Build history of the part. All positions in model axes, mm. Face numbers are marked on the shaded views. Give positions to 0.01 mm unless a question says otherwise; leave off trailing zeros. Order: outer loops, then holes, each group sorted by start corner. A loop starts at its lowest first (then second) coordinate and runs counter-clockwise, first axis right, second up. Notation, with made-up numbers: M 32.5,73.5 L 67.5,73.5 A28 cw 67.5,95.5 Z; hole C 14,68 d6. An arc over 180 degrees is marked long. One line per item, written item: value. Start each with the question number.
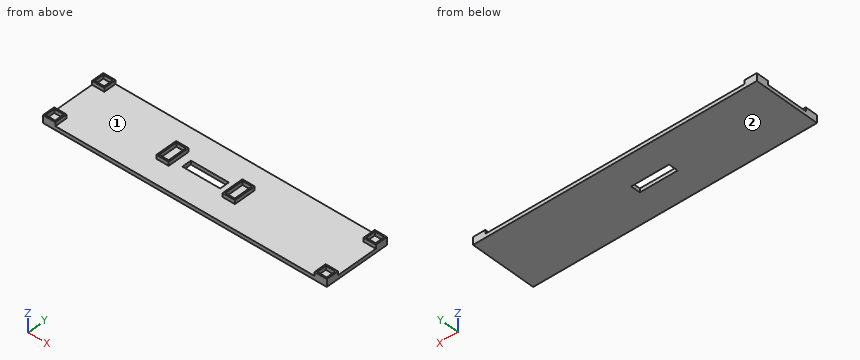
from build123d import *

# Parameters (mm, degrees)
SKICA1_W                 = 150
SKICA1_H                 = 35
P_IDAT_VYSUNUT_M2_DEPTH  = 2
SKICA2_W                 = 6.5
SKICA2_H                 = 11.5
SKICA2_W_2               = 5
SKICA2_H_2               = 10
P_IDAT_VYSUNUT_M3_DEPTH  = 2
SKICA3_W                 = 6.5
SKICA3_H                 = 6.5
SKICA3_W_2               = 5
SKICA3_H_2               = 5
P_IDAT_VYSUNUT_M4_DEPTH  = 2
SKICA4_W                 = 20
SKICA4_H                 = 5
ODEBRAT_VYSUNUT_M1_DEPTH = 2


with BuildPart() as part:
    # Skica1 → Přidat vysunutím2 (new body)
    with BuildSketch(Plane.XY):
        Rectangle(SKICA1_W, SKICA1_H)
    extrude(amount=P_IDAT_VYSUNUT_M2_DEPTH)

    # Skica2 → Přidat vysunutím3 (add)
    with BuildSketch(Plane.XY.offset(2)):
        with Locations((-22.5, 0)):
            Rectangle(SKICA2_W, SKICA2_H)
        with Locations((-22.5, 0)):
            Rectangle(SKICA2_W_2, SKICA2_H_2, mode=Mode.SUBTRACT)
        with Locations((12.5, 0)):
            Rectangle(SKICA2_W, SKICA2_H)
        with Locations((12.5, 0)):
            Rectangle(SKICA2_W_2, SKICA2_H_2, mode=Mode.SUBTRACT)
    extrude(amount=P_IDAT_VYSUNUT_M3_DEPTH)

    # Skica3 → Přidat vysunutím4 (add)
    with BuildSketch(Plane.XY.offset(2)):
        with Locations((-71.75, 14.25)):
            Rectangle(SKICA3_W, SKICA3_H)
        with Locations((-71.75, 14.25)):
            Rectangle(SKICA3_W_2, SKICA3_H_2, mode=Mode.SUBTRACT)
        with Locations((71.75, 14.25)):
            Rectangle(SKICA3_W, SKICA3_H)
        with Locations((71.75, 14.25)):
            Rectangle(SKICA3_W_2, SKICA3_H_2, mode=Mode.SUBTRACT)
        with Locations((-71.75, -14.25)):
            Rectangle(SKICA3_W, SKICA3_H)
        with Locations((-71.75, -14.25)):
            Rectangle(SKICA3_W_2, SKICA3_H_2, mode=Mode.SUBTRACT)
        with Locations((71.75, -14.25)):
            Rectangle(SKICA3_W, SKICA3_H)
        with Locations((71.75, -14.25)):
            Rectangle(SKICA3_W_2, SKICA3_H_2, mode=Mode.SUBTRACT)
    extrude(amount=P_IDAT_VYSUNUT_M4_DEPTH)

    # Skica4 → Odebrat vysunutím1 (cut)
    with BuildSketch(Plane.XY.offset(2)):
        with Locations((-5, 0)):
            Rectangle(SKICA4_W, SKICA4_H)
    extrude(amount=-ODEBRAT_VYSUNUT_M1_DEPTH, mode=Mode.SUBTRACT)


solid = part.part
1) Slice it at A-A (z = 3.25). State how many separate pieces and enclosed holes the cut face has, plus the area to 4 significant figures.
2) Drill centre lines: line 1 (X direction, y = 12, z = 2.3); line 2 (X direction, y = 0.5, z = 3.35); line 3 (X direction, y = -0.5, z = 0.8). Where is each one in solid material? Low to high.
3) Pull direction X, two halves, no side cores. Call the marked faces 1 and 2: pulls with the +X half, pulls with the -X half, needs draft (parallel to the pull), parting line crosses it, or undercut.
4) Slice it at D-D (x = 41). List the corners of the cut face in (y, z), plus the area to 3 significant figures.
5) Drop flat-ended pins along their axis: P1, Ø3, axis at x = -48.5, y = 8.5, coming from the +Z side; P2, Ø1, axis at x = -39, z = 3, coming from the -Y side. Give the stop position or say it passes through.
6) Slice it at B-B (y = 13). List the corners of the cut face in (x, z), plus the area to 3 significant figures.
7) Slice it at C-C (x = -22). List the corners of the cut face in (y, z).
Results list:
1. separate pieces: 6
1. enclosed holes: 6
1. area: 118.5 mm²
2. line 1: x = -75 to -74.25, -69.25 to -68.5, 68.5 to 69.25, 74.25 to 75
2. line 2: x = -25.75 to -25, -20 to -19.25, 9.25 to 10, 15 to 15.75
2. line 3: x = -75 to -15, 5 to 75
3. face 1: undercut
3. face 2: needs draft
4. outline: M -17.5,0 L 17.5,0 L 17.5,2 L -17.5,2 Z
4. area: 70.0 mm²
5. P1: stops at z = 2
5. P2: passes through
6. outline: M -75,0 L 75,0 L 75,4 L 74.25,4 L 74.25,2 L 69.25,2 L 69.25,4 L 68.5,4 L 68.5,2 L -68.5,2 L -68.5,4 L -69.25,4 L -69.25,2 L -74.25,2 L -74.25,4 L -75,4 Z
6. area: 306 mm²
7. outline: M -17.5,0 L 17.5,0 L 17.5,2 L 5.75,2 L 5.75,4 L 5,4 L 5,2 L -5,2 L -5,4 L -5.75,4 L -5.75,2 L -17.5,2 Z
